CAD build for the part. Positions are in the model's coordinates, mm. A direction names the side the tool comes from. Round coordinates to 2 decimals unless told otherwise and drop trailing zeros. Loops run counter-clockwise (first coordinate to the right, second up) from the corner with the lowest first, then second, coordinate; pieces in that order, holes last. Notation, with made-up numbers: M 77,15 L 125,15 A14 ccw 125,24 Z; hole C 16,7.5 d11. An arc over 180 degrees is marked long. Use one line per item in the form item = value.
from build123d import *

# Parameters (mm, degrees)
F0_W     = 112
F0_H     = 30
F0_R     = 3
F1_DEPTH = 3
F3_DEPTH = 25
F4_R     = 3
F5_DEPTH = 25


with BuildPart() as f1:
    # F0 (on Front) → F1 (new body)
    with BuildSketch(Plane.XZ):
        Rectangle(F0_W, F0_H)
        with Locations((-45.5, 8)):
            Circle(F0_R, mode=Mode.SUBTRACT)
    extrude(amount=F1_DEPTH)

    # F2 (on face) → F3 (cut)
    with BuildSketch(Plane.XZ.offset(3)):
        Polygon((-38, 4), (-38, 2), (-38, 0), (-31, 0), (-31, -7), (-29, -7), (-27, -7), (-27, 0), (-20, 0), (-20, 2), (-20, 4), (-27, 4), (-27, 11), (-29, 11), (-31, 11), (-31, 4), align=None)
    extrude(amount=-F3_DEPTH, mode=Mode.SUBTRACT)

    # F4 (on face) → F5 (cut)
    with BuildSketch(Plane.XZ.offset(3)):
        with Locations((30.1, 0)):
            Circle(F4_R)
        with BuildLine():
            ThreePointArc((43.25, 0), (40.25, 3), (37.25, 0))
            ThreePointArc((37.25, 0), (40.25, -3), (43.25, 0))
        make_face()
    extrude(amount=-F5_DEPTH, mode=Mode.SUBTRACT)


solid = f1.part
1. Cut at C-C on y = -0.45. Write the cut outline in (x, z).
Completed:
outline = M -56,-15 L 56,-15 L 56,15 L -56,15 Z; hole C -45.5,8 d6; hole M -38,0 L -31,0 L -31,-7 L -27,-7 L -27,0 L -20,0 L -20,4 L -27,4 L -27,11 L -31,11 L -31,4 L -38,4 Z; hole C 30.1,0 d6; hole C 40.25,0 d6
2. Cut at A-A on z = 8. Write the cut outline in (x, y).
Completed:
outline = M -56,-3 L -48.5,-3 L -48.5,0 L -56,0 Z; M -42.5,-3 L -31,-3 L -31,0 L -42.5,0 Z; M -27,-3 L 56,-3 L 56,0 L -27,0 Z
3. Cut at D-D on z = -5.5. Write the cut outline in (x, y).
Completed:
outline = M -56,-3 L -31,-3 L -31,0 L -56,0 Z; M -27,-3 L 56,-3 L 56,0 L -27,0 Z
4. Cut at B-B on x = 40.25. Write the cut outline in (y, z), and give its area (3 significant figures).
Completed:
outline = M -3,-15 L 0,-15 L 0,-3 L -3,-3 Z; M -3,3 L 0,3 L 0,15 L -3,15 Z
area = 72.0 mm2
5. Pull direction X, two halves, no side cores. Call faces 3 (the face through (43.247, -1.521, -0.132)), 4 (the face through (-1, -1, -15)), 5 (the face through (56, -1, 0)): +X half, -X half, draft (parallel to the pull), parting line (faces both ways), or undercut.
Completed:
face_3 = undercut
face_4 = draft
face_5 = +X half
6. Probe line 1 along Z through (x, y) = (30.1, -1.55); line 2 along Z through (x, y) = (-22, -1.25); line 3 along X through (y, z) = (-1.6, 1.5). List the from-to ranges inside material, lowest first. Write a range as from..to.
Completed:
line_1 = -15..-3, 3..15
line_2 = -15..0, 4..15
line_3 = -56..-38, -20..27.5, 32.7..37.65, 42.85..56
7. Tool access for faces 1 (the face through (-38, -2, 2)), 2 (the face through (-1, -1, 15)): list every direction of +Z, -Z, +X, -X, +Y, -Y with a clear straight run to the whole face (end or side of a thin tool).
Completed:
face_1 = +Y, -Y
face_2 = +Z, +X, -X, +Y, -Y
